Design review of the part built by this model. Coordinates are the model's own, in mm. A direction names the side the tool comes from. Round coordinates to 2 decimals unless told otherwise and drop trailing zeros. Loops run counter-clockwise (first coordinate to the right, second up) from the corner with the lowest first, then second, coordinate; pieces in that order, holes last. Notation, with made-up numbers: M 48,-20.75 L 70,-20.75 A12 cw 70,1.25 Z; hole C -28,67 d11. An arc over 180 degrees is marked long. Use a Markdown table: item, result.
from build123d import *

# Parameters (mm, degrees)
SKETCH2_W           = 60
SKETCH2_H           = 64
TOP_DEPTH           = 3.2
SKETCH3_R           = 1.5
ARDUINO_HOLES_DEPTH = 3.2
SKETCH5_R           = 1
BATTERY_CUT_DEPTH   = 3.2
SKETCH7_W           = 9.78
SKETCH7_H           = 3.18
FRICTION_FIT_DEPTH  = 10


with BuildPart() as part:
    # Sketch2 → Top (new body)
    with BuildSketch(Plane.XY):
        with Locations((-2.549375328, 23.639166253)):
            Rectangle(SKETCH2_W, SKETCH2_H)
    extrude(amount=TOP_DEPTH)

    # Sketch3 → Arduino Holes (cut)
    with BuildSketch(Plane.XY.offset(3.2)):
        with Locations((20.950624672, 2.339166253)):
            Circle(SKETCH3_R)
        with Locations((22.450624672, 50.639166253)):
            Circle(SKETCH3_R)
        with Locations((-29.849375328, 17.639166253)):
            Circle(SKETCH3_R)
        with Locations((-29.849375328, 45.539166253)):
            Circle(SKETCH3_R)
    extrude(amount=-ARDUINO_HOLES_DEPTH, mode=Mode.SUBTRACT)

    # Sketch5 → Battery Cut (cut)
    with BuildSketch(Plane(origin=(0, 0, 0), x_dir=(-1, 0, 0), z_dir=(0, 0, -1))):
        with Locations((-2.450624672, 35.639166253)):
            Circle(SKETCH5_R)
        with Locations((-16.200624672, 14.139166253)):
            Circle(SKETCH5_R)
        with Locations((11.299375328, 14.139166253)):
            Circle(SKETCH5_R)
    extrude(amount=-BATTERY_CUT_DEPTH, mode=Mode.SUBTRACT)

    # Sketch7 → Friction Fit (cut)
    with BuildSketch(Plane(origin=(0, 0, 0), x_dir=(-1, 0, 0), z_dir=(0, 0, -1))):
        with Locations((2.549375328, 54.049166253)):
            Rectangle(SKETCH7_W, SKETCH7_H)
        with Locations((2.549375328, -6.770833747)):
            Rectangle(SKETCH7_W, SKETCH7_H)
    extrude(amount=-FRICTION_FIT_DEPTH, mode=Mode.SUBTRACT)


solid = part.part
1. Insertion check: pin 1 (1 mm diameter, centred on x = -1.5, z = 2.5, fed in from -Y); pin 2 (1.6 mm diameter, centred on x = -0.5, z = 2, fed in from +Y). Each pin has a flat end and moves straight along its axis. Give the tip position at first contact, or say it passes through.
Check values:
| item | result |
|---|---|
| pin 1 | stops at y = -5.18 |
| pin 2 | stops at y = 52.46 |
2. Take a section at A-A on z = 1.7. Give the boundary of the cut face in (x, y).
Check values:
| item | result |
|---|---|
| outline | M -32.55,-8.36 L -7.44,-8.36 L -7.44,-5.18 L 2.34,-5.18 L 2.34,-8.36 L 27.45,-8.36 L 27.45,55.64 L 2.34,55.64 L 2.34,52.46 L -7.44,52.46 L -7.44,55.64 L -32.55,55.64 Z; hole C -29.85,17.64 d3; hole C -29.85,45.54 d3; hole C -11.3,14.14 d2; hole C 2.45,35.64 d2; hole C 16.2,14.14 d2; hole C 20.95,2.34 d3; hole C 22.45,50.64 d3 |
3. Wall thickness on line 1 along X through (y, z) = (35, 0.5); line 2 along X through (y, z) = (18, 2.7); line 3 along Y through (x, z) = (-5, 1.65): over which ranges is each line inside the solid? List them lowest first. Write a range as from..to.
Check values:
| item | result |
|---|---|
| line 1 | x = -32.55..1.68, 3.22..27.45 |
| line 2 | x = -32.55..-31.31, -28.39..27.45 |
| line 3 | y = -5.18..52.46 |
4. Take a section at B-B on x = 16. Give the boundary of the cut face in (y, z).
Check values:
| item | result |
|---|---|
| outline | M -8.36,0 L 13.16,0 L 13.16,3.2 L -8.36,3.2 Z; M 15.12,0 L 55.64,0 L 55.64,3.2 L 15.12,3.2 Z |
5. Machinability: for faces 1 (the face through (2.341, -7, 2)), 2 (the face through (-7.439, 54, 2)), 3 (the face through (-11.17, 15.13, 1.58)), which of the approach directions +Z, -Z, +X, -X, +Y, -Y give a long, thin tool a straight path to every point of the face, cutting with its end or side? Answer none if there is none.
Check values:
| item | result |
|---|---|
| face 1 | +Z, -Z, -Y |
| face 2 | +Z, -Z, +Y |
| face 3 | +Z, -Z |
6. Take a section at C-C on x = -3. Give the boundary of the cut face in (y, z).
Check values:
| item | result |
|---|---|
| outline | M -5.18,0 L 52.46,0 L 52.46,3.2 L -5.18,3.2 Z |
7. The part is to be moulded in two halves that separate along Y. For faces 4 (the face through (1.91, 36.48, 1.58)), 5 (the face through (27.451, 23, 2)), 6 (the face through (-2, -5.181, 2)), say which applies: pulls with the +Y half, pulls with the -Y half, needs draft (parallel to the pull), parting line crosses it, or undercut.
Check values:
| item | result |
|---|---|
| face 4 | undercut |
| face 5 | needs draft |
| face 6 | pulls with the -Y half |
